Work out the finished part from the listing and answer in its coordinate system (mm). Face numbers are marked on the shaded views. Coordinates: 2 decimals unless noted, no trailing zeros. Write each loop counter-clockwise with the first axis right and the second up, starting at its lowest first coordinate (ties: lowest second). Pieces come first, ordered by that corner, then holes. Notation, with made-up numbers: M 73.5,-31.75 L 113.5,-31.75 A10 cw 113.5,-19.75 Z; hole C -14,66.25 d1. An arc over 180 degrees is marked long. Use CSV: the item, a comma, the result in double quotes.
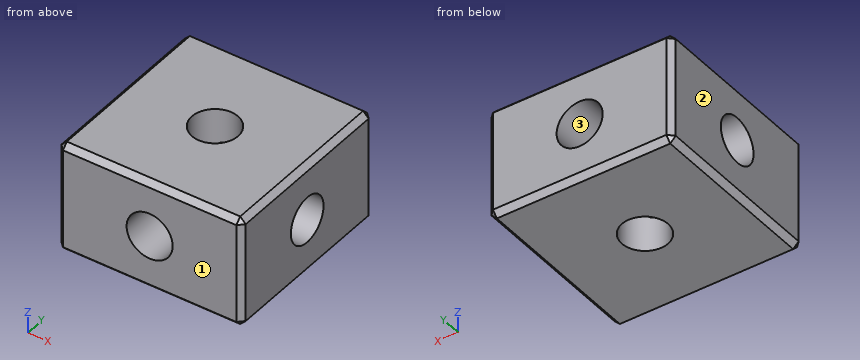
from build123d import *

# Parameters (mm, degrees)
SKETCH_1_W      = 10
SKETCH_1_H      = 10
EXTRUDE_1_DEPTH = 3
HOLE_WIZARD_1_D = 2.5
HOLE_WIZARD_2_D = 2.5
HOLE_WIZARD_3_D = 2.5
CHAMFER_1_SIZE  = 0.3


with BuildPart() as part:
    # 草图1 → 凸台-拉伸1 (new, symmetric)
    with BuildSketch(Plane.XY):
        Rectangle(SKETCH_1_W, SKETCH_1_H)
    extrude(amount=EXTRUDE_1_DEPTH, both=True)

    # 螺纹孔1 (through all)
    with Locations(Plane.XY.offset(3)):
        with Locations((0, 0)):
            Hole(HOLE_WIZARD_1_D / 2)

    # Hole Wizard 2 (through all)
    with Locations(Plane(origin=(5, 0, 0), x_dir=(0, 0, -1), z_dir=(1, 0, 0))):
        with Locations((0, 0)):
            Hole(HOLE_WIZARD_2_D / 2)

    # 螺纹孔3 (through all)
    with Locations(Plane(origin=(0, -5, 0), x_dir=(-1, 0, 0), z_dir=(0, -1, 0))):
        with Locations((0, 0)):
            Hole(HOLE_WIZARD_3_D / 2)

    # 倒角1
    chamfer_1_edges = [part.edges().sort_by_distance(p)[0] for p in [
        (-5, 0, 3),
        (0, -5, 3),
        (5, 0, 3),
        (0, -5, -3),
        (-5, 0, -3),
        (0, 5, -3),
        (5, 0, -3),
        (5, -5, 0),
        (-5, -5, 0),
        (-5, 5, 0),
        (5, 5, 0),
        (0, 5, 3),
    ]]
    chamfer(chamfer_1_edges, length=CHAMFER_1_SIZE)


solid = part.part
Item 1: Given pin 1 (2 mm diameter, centred on x = 0, y = 0, fed in from -Z); pin 2 (4 mm diameter, centred on x = 0, y = 1, fed in from +Z), each flat-ended and moving along its own axis, determine where each tip first touches the part or whether it passes through.
Answer:
pin 1,"passes through"
pin 2,"stops at z = 3"
Item 2: Consider probe 1 along Z at (x, y) = (0, -3.6); probe 2 along Y at (x, z) = (-3.4, 0). Determine where each line is inside the solid, lowest interval first.
Answer:
probe 1,"z = -3 to -1.25, 1.25 to 3"
probe 2,"y = -5 to -1.25, 1.25 to 5"
Item 3: For a pull along X with two mould halves and no side action, classify the marked faces 1, 2 and 3 as released by +X, released by -X, zero draft, split by the parting line, or undercut.
Answer:
face 1,"zero draft"
face 2,"released by -X"
face 3,"undercut"
Item 4: The part is cut by section A-A (y = 0). Write down the section's boundary in (x, z), then the cut area to 3 significant figures.
Answer:
outline,"M -5,-2.7 L -4.7,-3 L -1.25,-3 L -1.25,-1.25 L -5,-1.25 Z; M -5,1.25 L -1.25,1.25 L -1.25,3 L -4.7,3 L -5,2.7 Z; M 1.25,-3 L 4.7,-3 L 5,-2.7 L 5,-1.25 L 1.25,-1.25 Z; M 1.25,1.25 L 5,1.25 L 5,2.7 L 4.7,3 L 1.25,3 Z"
area,"26.1 mm2"
Item 5: The part is cut by section C-C (x = 2.5). Write down the section's boundary in (y, z), then the cut area to 3 significant figures.
Answer:
outline,"M -5,-2.7 L -4.7,-3 L 4.7,-3 L 5,-2.7 L 5,2.7 L 4.7,3 L -4.7,3 L -5,2.7 Z; hole C 0,0 d2.5"
area,"54.9 mm2"
